```python
from build123d import *

# Parameters (mm, degrees)
FILLET_R = 2


with BuildPart() as part:
    # Sketch → Revolution (revolve)
    with BuildSketch(Plane.XZ):
        Polygon((0, 0), (20, 0), (20, 40), (10, 40), (10, 45), (3, 45), (3, 55), (0, 55), align=None)
    revolve(axis=Axis((0, 0, 0), (0, 0, 1)))

    # Fillet
    fillet_edges = [part.edges().sort_by_distance(p)[0] for p in [
        (-20, 0, 0),
    ]]
    fillet(fillet_edges, radius=FILLET_R)


solid = part.part
```
Work out the finished part from the listing and answer in its coordinate system (mm). A direction names the side the tool comes from. Round coordinates to 2 decimals unless told otherwise and drop trailing zeros. Write each loop counter-clockwise with the first axis right and the second up, starting at its lowest first coordinate (ties: lowest second). Pieces come first, ordered by that corner, then holes.
1) A cutting plane is placed at C-C on z = 21. Determine the outline of the cut face in (x, y).
2) Consider probe 1 along Z at (x, y) = (10.5, 5); probe 2 along Z at (x, y) = (8, -5); probe 3 along X at (y, z) = (-10.5, 36). Determine where each line is inside the solid, lowest interval first.
3) A cutting plane is placed at D-D on z = 48.5. Determine the outline of the cut face in (x, y), and give its area (3 significant figures).
4) Which of the six approach directions +Z, -Z, +X, -X, +Y, -Y give full straight-line access (tool end or side, diameter ignored) to faces 4 (the face through (-2.17, -9.76, 42.54)), 5 (the face through (-4.336, -19.524, 21.266))?
5) Determine the mould class of faces 1 (the face through (-5, 9, 40)), 2 (the face through (0, 0, 0)), 3 (the face through (-3, 0, 50)) for opening direction Z: pulls with the +Z half, pulls with the -Z half, needs draft (parallel to the pull), parting line crosses it, or undercut.
6) Flat-ended cylindrical pins translate along their axes: P1, Ø10, axis at y = -11.5, z = 34, coming from the -X side; P2, Ø6, axis at x = 13.5, y = -16, coming from the +Z side; P3, Ø5, axis at y = 13.5, z = 35, coming from the -X side. Find the tip coordinate at first contact, or state that the pin passes through.
7) A cutting plane is placed at A-A on x = 0. Determine the outline of the cut face in (y, z), and give its area (3 significant figures).
Entries:
1. outline: circle Ø40 at (0, 0)
2. probe 1: z = 0 to 40
2. probe 2: z = 0 to 45
2. probe 3: x = -17.02 to 17.02
3. outline: circle Ø6 at (0, 0)
3. area: 28.3 mm2
4. face 4: +Z
4. face 5: +Z, -Z
5. face 1: pulls with the +Z half
5. face 2: pulls with the -Z half
5. face 3: needs draft
6. P1: stops at x = -18.91
6. P2: stops at z = 40
6. P3: stops at x = -16.7
7. outline: (-20, 2) arc R2 ccw to (-18, 0) - (18, 0) arc R2 ccw to (20, 2) - (20, 40) - (10, 40) - (10, 45) - (3, 45) - (3, 55) - (-3, 55) - (-3, 45) - (-10, 45) - (-10, 40) - (-20, 40) - close
7. area: 1,760 mm2
